```python
from build123d import *

# Parameters (mm, degrees)
F0_W     = 25.4
F0_H     = 254
F0_W_2   = 508
F0_H_2   = 25.4
F1_DEPTH = 914.4
F2_W     = 914.4
F2_H     = 508
F3_DEPTH = 50.8
F4_W     = 508
F4_H     = 127
F4_H_2   = 152.4
F4_H_3   = 177.8
F5_DEPTH = 127
F6_R     = 12.7


with BuildPart() as f1:
    # F0 (on Top) → F1 (new body)
    with BuildSketch(Plane.XY):
        Polygon((-279.4, 127), (-254, 127), (-254, 152.4), (-254, 177.8), (-304.8, 177.8), (-304.8, 127), align=None)
        Polygon((-254, -177.8), (-254, -152.4), (-254, -127), (-279.4, -127), (-304.8, -127), (-304.8, -177.8), align=None)
        Polygon((254, -152.4), (254, -177.8), (304.8, -177.8), (304.8, -127), (279.4, -127), (254, -127), align=None)
        Polygon((254, 152.4), (254, 127), (279.4, 127), (304.8, 127), (304.8, 177.8), (254, 177.8), align=None)
        with Locations((-266.7, 0)):
            Rectangle(F0_W, F0_H)
        with Locations((0, 139.7)):
            Rectangle(F0_W_2, F0_H_2)
        with Locations((266.7, 0)):
            Rectangle(F0_W, F0_H)
        with Locations((0, -139.7)):
            Rectangle(F0_W_2, F0_H_2)
    extrude(amount=F1_DEPTH)

    # F2 (on face) → F3 (join)
    with BuildSketch(Plane.XY.offset(914.4)):
        Rectangle(F2_W, F2_H)
    extrude(amount=F3_DEPTH)

    # F4 (on face) → F5 (cut)
    with BuildSketch(Plane.XZ.offset(152.4)):
        with Locations((0, 723.9)):
            Rectangle(F4_W, F4_H)
        with Locations((0, 508)):
            Rectangle(F4_W, F4_H_2)
        with Locations((0, 266.7)):
            Rectangle(F4_W, F4_H_3)
    extrude(amount=-F5_DEPTH, mode=Mode.SUBTRACT)

    # F6
    f6_edges = [f1.edges().sort_by_distance(p)[0] for p in [
        (457.2, 0, 965.2),
        (0, -254, 965.2),
        (-457.2, 0, 965.2),
        (0, 254, 965.2),
        (457.2, -254, 939.8),
        (-457.2, -254, 939.8),
        (457.2, 254, 939.8),
        (-457.2, 254, 939.8),
        (304.8, -177.8, 457.2),
        (-304.8, -177.8, 457.2),
        (304.8, 177.8, 457.2),
        (-304.8, 177.8, 457.2),
    ]]
    fillet(f6_edges, radius=F6_R)


solid = f1.part
```
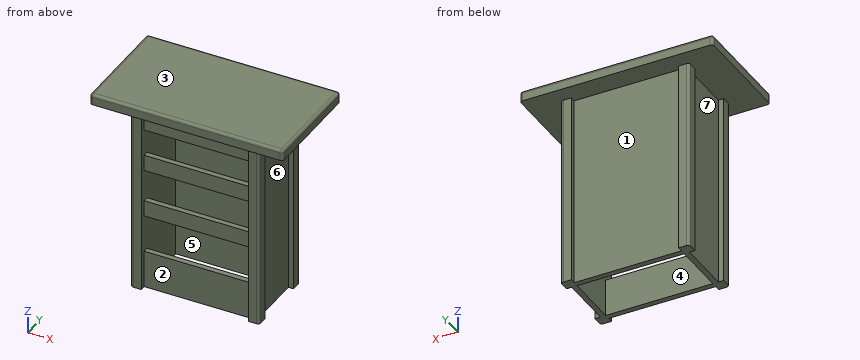
Can you work these out from the model? Positions are in its coordinate system, mm. Face numbers are marked on the shaded views. A direction names the side the tool comes from. Coordinates: 2 decimals unless noted, no trailing zeros. Order: outer loops, then holes, each group sorted by start corner. A loop starts at its lowest first (then second) coordinate and runs counter-clockwise, first axis right, second up. Notation, with made-up numbers: (21, 3.5) - (66, 3.5) arc R14 ccw to (66, 14.5) - close; hole circle Ø5 at (12.5, 54). An arc over 180 degrees is marked (long way). Answer in a Markdown table with one row per item.
1. Suppose I cut it at A-A (x = -20). Please give me the cut outline in (y, z), and give its area (3 significant figures).
Reply:
| item | result |
|---|---|
| outline | (-254, 914.4) - (-152.4, 914.4) - (-152.4, 787.4) - (-127, 787.4) - (-127, 914.4) - (127, 914.4) - (127, 0) - (152.4, 0) - (152.4, 914.4) - (254, 914.4) - (254, 952.5) arc R12.7 ccw to (241.3, 965.2) - (-241.3, 965.2) arc R12.7 ccw to (-254, 952.5) - close; (-152.4, 0) - (-127, 0) - (-127, 177.8) - (-152.4, 177.8) - close; (-152.4, 355.6) - (-127, 355.6) - (-127, 431.8) - (-152.4, 431.8) - close; (-152.4, 584.2) - (-127, 584.2) - (-127, 660.4) - (-152.4, 660.4) - close |
| area | 60,600 mm^2 |
2. For pin 1 (20.5 mm diameter, centred on x = 290, z = 655, fed in from -Y); pin 2 (3 mm diameter, centred on x = 271.5, z = 404, fed in from +Y); pin 3 (2 mm diameter, centred on y = 80.5, z = 833.5, fed in from -X); pin 4 (2 mm diameter, centred on x = -307.5, z = 191.5, fed in from +Y), each with a flat end and sliding along its axis, tell me the tip position at first contact or that it passes through.
Reply:
| item | result |
|---|---|
| pin 1 | stops at y = -177.8 |
| pin 2 | stops at y = 177.8 |
| pin 3 | stops at x = -279.4 |
| pin 4 | passes through |
3. Suppose I cut it at C-C (z = 812). Please give me the cut outline in (x, y).
Reply:
| item | result |
|---|---|
| outline | (-304.8, -165.1) arc R12.7 ccw to (-292.1, -177.8) - (-254, -177.8) - (-254, -152.4) - (254, -152.4) - (254, -177.8) - (292.1, -177.8) arc R12.7 ccw to (304.8, -165.1) - (304.8, -127) - (279.4, -127) - (279.4, 127) - (304.8, 127) - (304.8, 165.1) arc R12.7 ccw to (292.1, 177.8) - (254, 177.8) - (254, 152.4) - (-254, 152.4) - (-254, 177.8) - (-292.1, 177.8) arc R12.7 ccw to (-304.8, 165.1) - (-304.8, 127) - (-279.4, 127) - (-279.4, -127) - (-304.8, -127) - close; hole (-254, -127) - (254, -127) - (254, 127) - (-254, 127) - close |
4. Suppose I cut it at D-D (z = 226.5). Please give me the cut outline in (x, y).
Reply:
| item | result |
|---|---|
| outline | (-304.8, -165.1) arc R12.7 ccw to (-292.1, -177.8) - (-254, -177.8) - (-254, 127) - (254, 127) - (254, -177.8) - (292.1, -177.8) arc R12.7 ccw to (304.8, -165.1) - (304.8, -127) - (279.4, -127) - (279.4, 127) - (304.8, 127) - (304.8, 165.1) arc R12.7 ccw to (292.1, 177.8) - (254, 177.8) - (254, 152.4) - (-254, 152.4) - (-254, 177.8) - (-292.1, 177.8) arc R12.7 ccw to (-304.8, 165.1) - (-304.8, 127) - (-279.4, 127) - (-279.4, -127) - (-304.8, -127) - close |
5. For the marked faces 1, 2, 3 and 4, which set-ups out of +Z, -Z, +X, -X, +Y, -Y let a thin tool reach every point of the face, with its end or its side?
Reply:
| item | result |
|---|---|
| face 1 | -Z, +Y |
| face 2 | -Z, -Y |
| face 3 | +Z, +X, -X, +Y, -Y |
| face 4 | -Z |
6. If I drill on line 1 along Z through (x, y) = (-34.5, -147.5); line 2 along Y through (x, z) = (251, 609); line 3 along X through (y, z) = (-125, 236), over which ranges is the centre line in solid material (lowest first)?
Reply:
| item | result |
|---|---|
| line 1 | z = 0 to 177.8, 355.6 to 431.8, 584.2 to 660.4, 787.4 to 965.2 |
| line 2 | y = -152.4 to -127, 127 to 152.4 |
| line 3 | x = -279.4 to -254, 254 to 279.4 |
7. Suppose I cut it at B-B (y = 16). Please give me the cut outline in (x, z), and give its area (3 significant figures).
Reply:
| item | result |
|---|---|
| outline | (-457.2, 914.4) - (-279.4, 914.4) - (-279.4, 0) - (-254, 0) - (-254, 914.4) - (254, 914.4) - (254, 0) - (279.4, 0) - (279.4, 914.4) - (457.2, 914.4) - (457.2, 952.5) arc R12.7 ccw to (444.5, 965.2) - (-444.5, 965.2) arc R12.7 ccw to (-457.2, 952.5) - close |
| area | 92,800 mm^2 |
8. If we mould it in two halves opening along X, with no side actions, what happens to the marked faces 5, 6 and 7? For each: pulls with the +X half, pulls with the -X half, needs draft (parallel to the pull), parting line crosses it, or undercut.
Reply:
| item | result |
|---|---|
| face 5 | undercut |
| face 6 | pulls with the +X half |
| face 7 | pulls with the -X half |
